Here's the drawing with two shaded views (mm, measured from the low corner). I have some questions. A direction names the side the tool comes from. Round coordinates to 2 decimals unless told otherwise and drop trailing zeros. Loops run counter-clockwise (first coordinate to the right, second up) from the corner with the lowest first, then second, coordinate; pieces in that order, holes last.
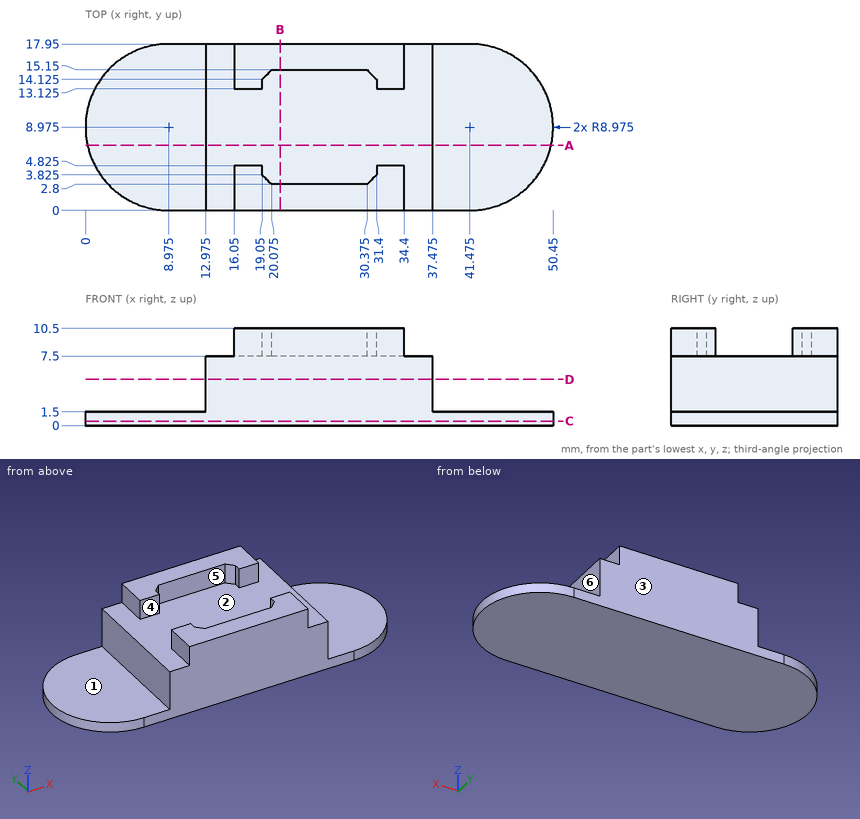
Item 1: If I drill on line 1 along X through (y, z) = (1.5, 9.5); line 2 along Z through (x, y) = (14, 1.25); line 3 along X through (y, z) = (10.5, 4.25) (3 decimals), over which ranges is the centre line in solid material (lowest first)?
Results list:
line 1: x = 16.05 to 34.4
line 2: z = 0 to 7.5
line 3: x = 12.975 to 37.475
Item 2: Will these pins go through, and if not, where does the flat tip stop? pin 1 (1.5 mm diameter, centred on y = 15, z = 9, fed in from +X); pin 2 (10.5 mm diameter, centred on x = 45.5, y = 10.5, fed in from +Z); pin 3 (0.9 mm diameter, centred on y = 16, z = 9, fed in from -X); pin 4 (3.5 mm diameter, centred on x = 18, z = 9, fed in from -Y).
Results list:
pin 1: stops at x = 34.4
pin 2: stops at z = 1.5
pin 3: stops at x = 16.05
pin 4: stops at y = 0
Item 3: If we section it at B-B, the plane x = 21: Please give me the cut outline in (y, z).
Results list:
outline: (0, 0) - (17.95, 0) - (17.95, 10.5) - (15.15, 10.5) - (15.15, 7.5) - (2.8, 7.5) - (2.8, 10.5) - (0, 10.5) - close
Item 4: If we section it at A-A, the plane y = 7: Please give me the cut outline in (x, z) (3 decimals).
Results list:
outline: (0.22, 0) - (50.23, 0) - (50.23, 1.5) - (37.475, 1.5) - (37.475, 7.5) - (12.975, 7.5) - (12.975, 1.5) - (0.22, 1.5) - close
Item 5: If we section it at C-C, the plane z = 0.5: Please give me the cut outline in (x, y) (3 decimals), then the cut area to 3 significant figures.
Results list:
outline: (8.975, 0) - (41.475, 0) arc R8.975 ccw to (41.475, 17.95) - (8.975, 17.95) arc R8.975 ccw to start
area: 836 mm2
Item 6: If we section it at D-D, the plane z = 5: Please give me the cut outline in (x, y) (3 decimals), then the cut area to 3 significant figures.
Results list:
outline: (12.975, 0) - (37.475, 0) - (37.475, 17.95) - (12.975, 17.95) - close
area: 440 mm2
Item 7: For the marked faces 4, 5 and 6, which set-ups out of +Z, -Z, +X, -X, +Y, -Y let a thin tool reach every point of the face, with its end or its side?
Results list:
face 4: +Z, +X, -X
face 5: +Z
face 6: +Z, +X, +Y, -Y
Item 8: We'd pull the mould along Y, two halves only. Please class the marked faces 1, 2 and 3: released by +Y, released by -Y, zero draft, split by the parting line, or undercut.
Results list:
face 1: zero draft
face 2: undercut
face 3: released by +Y
